Study the drawing (mm; zero at the part's minimum x, y, z) and answer. A direction names the side the tool comes from. Coordinates: 2 decimals unless noted, no trailing zeros. Loops run counter-clockwise (first coordinate to the right, second up) from the corner with the lowest first, then second, coordinate; pieces in that order, holes last. Notation, with made-up numbers: (66.5, -28) - (95.5, -28) arc R25 ccw to (95.5, -15) - close; hole circle Ø3 at (78, -16.75). An arc over 180 degrees is marked (long way). Write each question's results on one line, items separated by ' | '. Start each with the question number.
(1) Find section C-C on z = 60. Determine the outline of the cut face in (x, y), then the cut area to 3 significant figures.
(2) Find section A-A on y = 60. Determine the outline of the cut face in (x, z), then the cut area to 3 significant figures.
(3) Consider line 1 (Y direction, x = 19, z = 60); line 2 (X direction, y = 44.5, z = 25); line 3 (Y direction, x = 8.5, z = 14). Determine where each line is inside the solid, lowest interval first. Write a range as from..to.
(4) Determine the mould class of the marked faces 1, 2, 3 and 4 for opening direction Y: released by +Y, released by -Y, zero draft, split by the parting line, or undercut.
(5) Find section B-B on x = 36. Determine the outline of the cut face in (y, z).
(6) For the marked faces 5 and 6, determine the directions among +Z, -Z, +X, -X, +Y, -Y from which every point of the face is accessible in a straight line to the end or side of a thin tool.
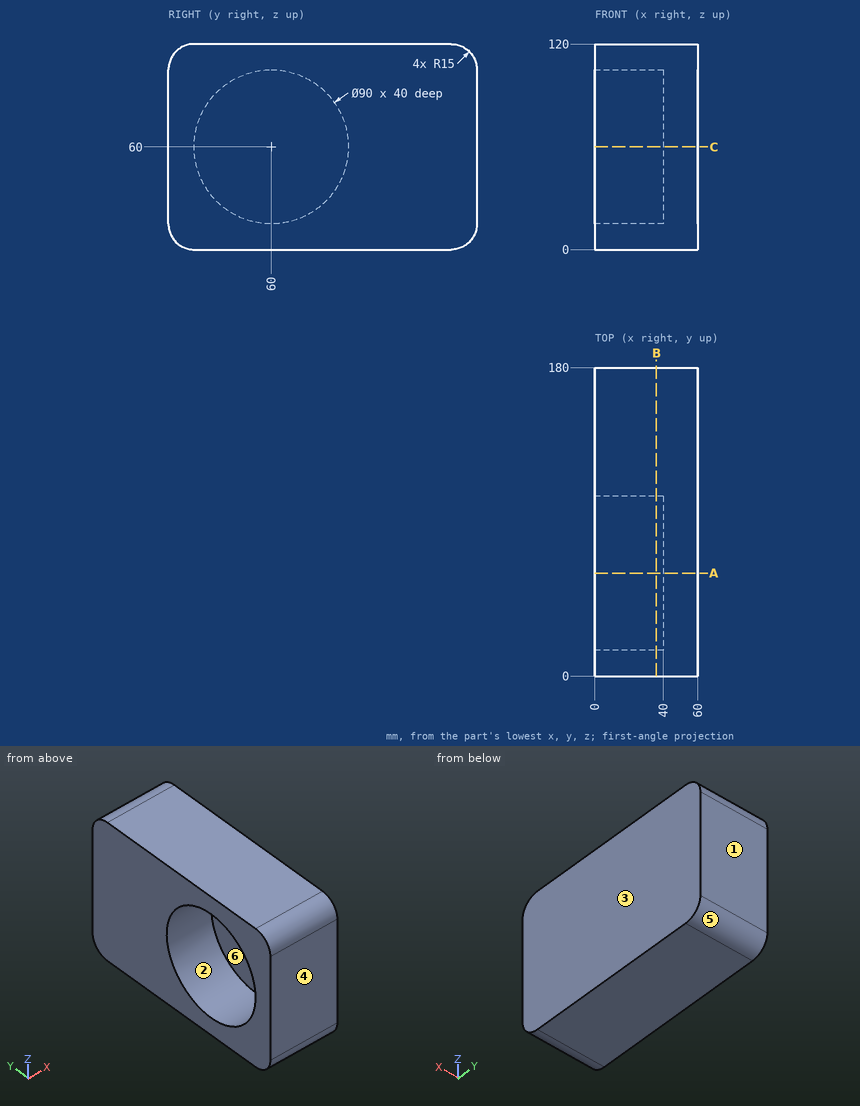
Values:
1) outline: (0, 0) - (60, 0) - (60, 180) - (0, 180) - (0, 105) - (40, 105) - (40, 15) - (0, 15) - close | area: 7,200 mm²
2) outline: (0, 0) - (60, 0) - (60, 120) - (0, 120) - (0, 105) - (40, 105) - (40, 15) - (0, 15) - close | area: 3,600 mm²
3) line 1: y = 0..15, 105..180 | line 2: x = 40..60 | line 3: y = 0.03..179.97
4) face 1: released by +Y | face 2: undercut | face 3: zero draft | face 4: released by -Y
5) outline: (0, 15) arc R15 ccw to (15, 0) - (165, 0) arc R15 ccw to (180, 15) - (180, 105) arc R15 ccw to (165, 120) - (15, 120) arc R15 ccw to (0, 105) - close; hole circle Ø90 at (60, 60)
6) face 5: -Z, +X, -X, +Y | face 6: -X
